The listing builds one solid part. Answer for the finished solid, in the listing's coordinates (mm). Face numbers are marked on the shaded views. A direction names the side the tool comes from. Round coordinates to 2 decimals unless told otherwise and drop trailing zeros. Loops run counter-clockwise (first coordinate to the right, second up) from the corner with the lowest first, then second, coordinate; pieces in that order, holes last. Notation, with made-up numbers: (5.25, -15) - (17.25, -15) arc R11 cw to (17.25, 1) - close; hole circle Ø7 at (-9.5, 68). An arc over 180 degrees is marked (long way). One line per item, written item: value.
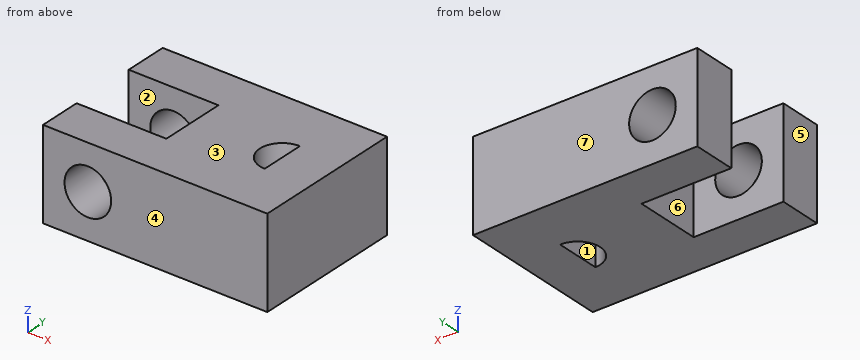
```python
from build123d import *

# Parameters (mm, degrees)
SKETCH1_W           = 31.75
SKETCH1_H           = 21.59
BOSS_EXTRUDE1_DEPTH = 12.7
SKETCH2_W           = 12.7
SKETCH2_H           = 9.398
CUT_EXTRUDE1_DEPTH  = 12.954
SKETCH3_R           = 3.302
CUT_EXTRUDE2_DEPTH  = 25.4
CUT_EXTRUDE3_DEPTH  = 31.75


with BuildPart() as part:
    # Sketch1 → Boss-Extrude1 (new body)
    with BuildSketch(Plane.XY):
        with Locations((15.875, 10.795)):
            Rectangle(SKETCH1_W, SKETCH1_H)
    extrude(amount=BOSS_EXTRUDE1_DEPTH)

    # Sketch2 → Cut-Extrude1 (cut)
    with BuildSketch(Plane.XY.offset(12.7)):
        with Locations((6.35, 10.763108956)):
            Rectangle(SKETCH2_W, SKETCH2_H)
    extrude(amount=-CUT_EXTRUDE1_DEPTH, mode=Mode.SUBTRACT)

    # Sketch3 → Cut-Extrude2 (cut)
    with BuildSketch(Plane.XZ):
        with Locations(Location((6.35, 6.35, 0), (0, 0, 270))):
            Circle(SKETCH3_R)
    extrude(amount=-CUT_EXTRUDE2_DEPTH, mode=Mode.SUBTRACT)

    # Sketch5 → Cut-Extrude3 (cut)
    with BuildSketch(Plane.XY.offset(12.7)):
        with BuildLine():
            Line((25.4, 13.97), (25.4, 7.62))
            ThreePointArc((25.4, 7.62), (22.225, 10.795), (25.4, 13.97))
        make_face()
    extrude(amount=-CUT_EXTRUDE3_DEPTH, mode=Mode.SUBTRACT)


solid = part.part
```
1) For the marked faces 1, 2 and 3, determine the directions among +Z, -Z, +X, -X, +Y, -Y from which every point of the face is accessible in a straight line to the end or side of a thin tool.
Final values:
face 1: +Z, -Z
face 2: +Z, -Z, -X
face 3: +Z, +X, -X, +Y, -Y
2) A cutting plane is placed at D-D on y = 13.5. Give the vertices of the cut face in (x, z).
Final values:
outline: (12.7, 0) - (23.74, 0) - (23.74, 12.7) - (12.7, 12.7) - close; (25.4, 0) - (31.75, 0) - (31.75, 12.7) - (25.4, 12.7) - close
3) Each of these flat-tipped pins is pushed along its axis until it touches: pin 1 Ø1 at (y, z) = (16.5, 4) entering from -X; pin 2 Ø4.5 at (y, z) = (12, 8) entering from -X; pin 3 Ø5.5 at (x, z) = (6.35, 6.35) entering from -Y. Where does it stop, or does it pass through?
Final values:
pin 1: x = 0
pin 2: x = 12.7
pin 3: through
4) A cutting plane is placed at A-A on x = 6.35. Give the vertices of the cut face in (y, z), and give its area (3 significant figures).
Final values:
outline: (0, 0) - (6.06, 0) - (6.06, 3.05) - (0, 3.05) - close; (0, 9.65) - (6.06, 9.65) - (6.06, 12.7) - (0, 12.7) - close; (15.46, 0) - (21.59, 0) - (21.59, 3.05) - (15.46, 3.05) - close; (15.46, 9.65) - (21.59, 9.65) - (21.59, 12.7) - (15.46, 12.7) - close
area: 74.3 mm2
5) For a pull along Y with two mould halves and no side action, classify the marked faces 4, 5, 6 and 7 as released by +Y, released by -Y, zero draft, split by the parting line, or undercut.
Final values:
face 4: released by -Y
face 5: zero draft
face 6: undercut
face 7: released by +Y
6) Consider L1, parallel to X at y = 1.5, z = 6.35; L2, parallel to Y at x = 12, z = 6.75. Determine where each line is inside the solid, lowest interval first.
Final values:
L1: 0 to 3.05, 9.65 to 31.75
L2: 0 to 6.06, 15.46 to 21.59
7) A cutting plane is placed at C-C on y = 1.5. Give the vertices of the cut face in (x, z).
Final values:
outline: (0, 0) - (31.75, 0) - (31.75, 12.7) - (0, 12.7) - close; hole circle Ø6.6 at (6.35, 6.35)
8) A cutting plane is placed at B-B on z = 6.35. Give the vertices of the cut face in (x, y) (3 decimals), and give its area (3 significant figures).
Final values:
outline: (0, 0) - (3.048, 0) - (3.048, 6.064) - (0, 6.064) - close; (0, 15.462) - (3.048, 15.462) - (3.048, 21.59) - (0, 21.59) - close; (9.652, 0) - (31.75, 0) - (31.75, 21.59) - (9.652, 21.59) - (9.652, 15.462) - (12.7, 15.462) - (12.7, 6.064) - (9.652, 6.064) - close; hole (25.4, 7.62) - (25.4, 13.97) arc R3.175 ccw to start
area: 470 mm2
